```python
from build123d import *

# Parameters (mm, degrees)
SKETCH1_R               = 4.765
BOSS_EXTRUDE1_DEPTH     = 9.525
CUT_EXTRUDE1_DEPTH      = 12.667736499
CUT_EXTRUDE1_DEPTH_BACK = 12.667736499
SKETCH2_R               = 3.43
CHAMFER1_SIZE           = 0.76


with BuildPart() as part:
    # Sketch1 → Boss-Extrude1 (new, symmetric)
    with BuildSketch(Plane.XY):
        with Locations(Location((0, 0, 0), (0, 0, 180))):
            Circle(SKETCH1_R)
    extrude(amount=BOSS_EXTRUDE1_DEPTH, both=True)

    # Sketch2 → Cut-Extrude1 (cut, two sides: drawn at the far end of the back side and taken through both)
    with BuildSketch(Plane(origin=(0, 0, 0), x_dir=(1, 0, 0), z_dir=(0, 1, 0)).offset(-CUT_EXTRUDE1_DEPTH_BACK)):
        with Locations(Location((-0.125, 0, 0), (0, 0, 270))):
            Circle(SKETCH2_R)
    extrude(amount=CUT_EXTRUDE1_DEPTH + CUT_EXTRUDE1_DEPTH_BACK, mode=Mode.SUBTRACT)

    # Chamfer1
    chamfer1_edges = [part.edges().sort_by_distance(p)[0] for p in [
        (4.765, 0, -9.525),
        (4.765, 0, 9.525),
    ]]
    chamfer(chamfer1_edges, length=CHAMFER1_SIZE)


solid = part.part
```
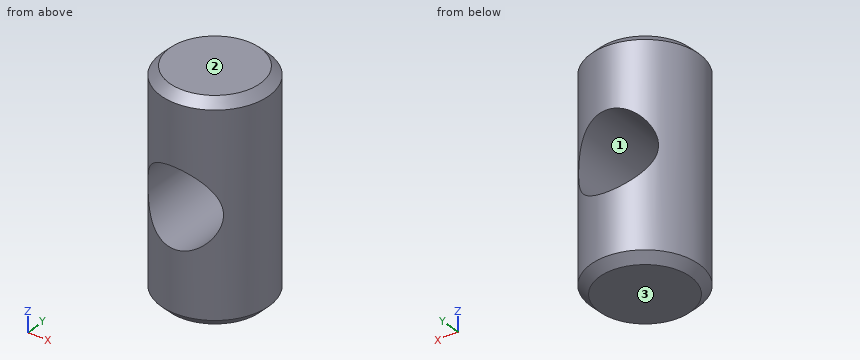
Part model, mm, in its own coordinate system. Face numbers are marked on the shaded views. Give positions to 0.01 mm unless a question says otherwise; leave off trailing zeros. Order: outer loops, then holes, each group sorted by start corner. A loop starts at its lowest first (then second) coordinate and runs counter-clockwise, first axis right, second up. Notation, with made-up numbers: (-17, 21.25) - (-2, 21.25) arc R29 ccw to (-2, 54.25) - close; hole circle Ø11 at (60, -22). An arc over 180 degrees is marked (long way). Use one line per item in the form item = value.
Item 1: Probe probe 1 along X at (y, z) = (2.5, 1.75); probe 2 along X at (y, z) = (1.5, -0.25); probe 3 along Z at (x, y) = (2.5, 0.75) (3 decimals). List the from-to ranges inside material, lowest first. Write a range as from..to.
Solution:
probe_1 = -4.06..-3.07, 2.82..4.06
probe_2 = -4.52..-3.55, 3.3..4.52
probe_3 = -9.525..-2.208, 2.208..9.525
Item 2: Slice it at C-C on z = 0. Give the cut face in (x, y) (3 decimals), and give its area (3 significant figures).
Solution:
outline = (-3.555, -3.173) - (-3.555, 3.173) arc R4.765 ccw to start; (3.305, -3.433) arc R4.765 ccw to (3.305, 3.433) - close
area = 12.2 mm2
Item 3: Two-plate mould, pull along Z, no slides. Class the marked faces 1, 2 and 3: released by +Z, released by -Z, zero draft, split by the parting line, or undercut.
Solution:
face_1 = undercut
face_2 = released by +Z
face_3 = released by -Z
Item 4: Slice it at A-A on y = 0. Give the cut face in (x, z) (3 decimals).
Solution:
outline = (-4.765, -8.765) - (-4.005, -9.525) - (4.005, -9.525) - (4.765, -8.765) - (4.765, 8.765) - (4.005, 9.525) - (-4.005, 9.525) - (-4.765, 8.765) - close; hole circle Ø6.86 at (-0.125, 0)
Item 5: Pin check, flat tips, straight feed: pin 1 Ø4 at (x, z) = (3, 6.5) entering from +Y; pin 2 Ø2 at (x, z) = (2.5, -5) entering from +Y; pin 3 Ø1.5 at (x, z) = (-1, 3.5) entering from -Y. Stop position of each tip, or through.
Solution:
pin_1 = 4.66
pin_2 = 4.52
pin_3 = -4.76
Item 6: Slice it at B-B on z = 6.75. Give the cut face in (x, y) (3 decimals).
Solution:
outline = circle Ø9.53 at (0, 0)
